Source: three-view drawing plus pictorial views. Frame: mm from the lowest corner of the part. A direction names the side the tool comes from. Coordinates: 2 decimals unless noted, no trailing zeros. Loops run counter-clockwise (first coordinate to the right, second up) from the corner with the lowest first, then second, coordinate; pieces in that order, holes last. Notation, with made-up numbers: (-5.5, 77.25) - (43.5, 77.25) arc R37 ccw to (43.5, 114.25) - close; hole circle Ø6 at (-23, -3.75). An arc over 180 degrees is marked (long way). Return JSON: item names as keys, results as strings.
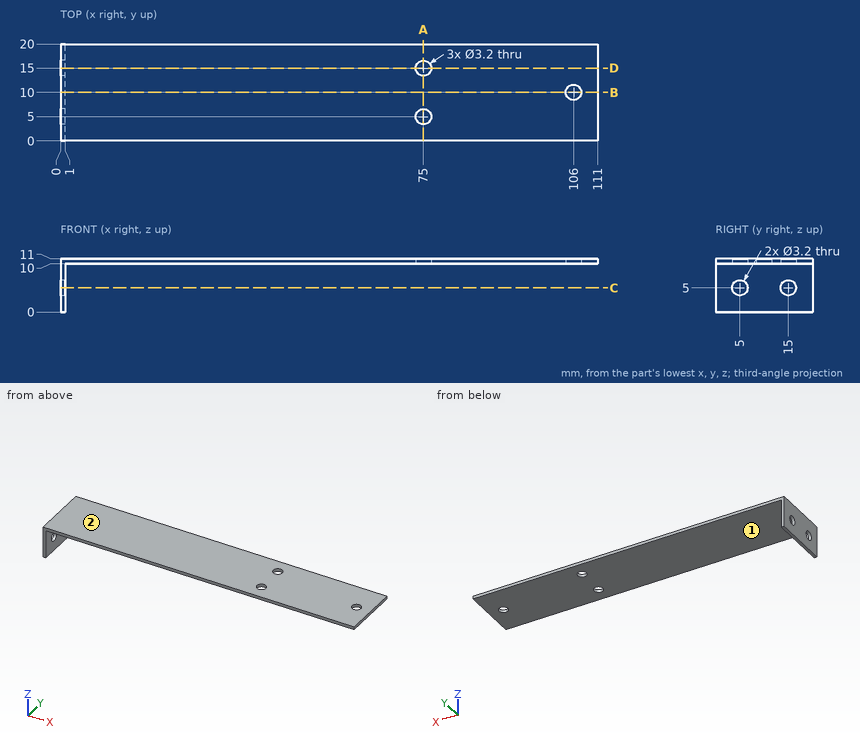
Item 1: Section query C-C, the plane z = 5. Return loops of the section in (x, y), and give its area (3 significant figures).
Worked out:
{"outline": "(0, 0) - (1, 0) - (1, 3.4) - (0, 3.4) - close; (0, 6.6) - (1, 6.6) - (1, 13.4) - (0, 13.4) - close; (0, 16.6) - (1, 16.6) - (1, 20) - (0, 20) - close", "area": "13.6 mm^2"}
Item 2: Reachability of the marked faces 1 and 2 from +Z, -Z, +X, -X, +Y, -Y: full face, straight path, thin tool, end or side. Return the list, or none.
Worked out:
{"face 1": "-Z, +X, +Y, -Y", "face 2": "+Z, +X, -X, +Y, -Y"}
Item 3: Ray query, probe 1 along Y at (x, z) = (0.45, 5); probe 2 along Y at (x, z) = (106, 10.2); probe 3 along X at (y, z) = (10, 10.7). Return the intervals inside material, ascending. Write a range as from..to.
Worked out:
{"probe 1": "0..3.4, 6.6..13.4, 16.6..20", "probe 2": "0..8.4, 11.6..20", "probe 3": "0..104.4, 107.6..111"}
Item 4: First-contact query: pin 1 Ø5 at (y, z) = (14.5, 6) entering from +X; pin 2 Ø4 at (x, y) = (12, 5.5) entering from -Z; pin 3 Ø3 at (x, y) = (75, 5) entering from -Z. Flat tips, straight axial feed; report the tip coordinate or a pass-through.
Worked out:
{"pin 1": "x = 1", "pin 2": "z = 10", "pin 3": "through"}
Item 5: Section query D-D, the plane y = 15. Return loops of the section in (x, z).
Worked out:
{"outline": "(0, 0) - (1, 0) - (1, 3.4) - (0, 3.4) - close; (0, 6.6) - (1, 6.6) - (1, 10) - (73.4, 10) - (73.4, 11) - (0, 11) - close; (76.6, 10) - (111, 10) - (111, 11) - (76.6, 11) - close"}
Item 6: Section query A-A, the plane x = 75. Return loops of the section in (y, z), and give its area (3 significant figures).
Worked out:
{"outline": "(0, 10) - (3.4, 10) - (3.4, 11) - (0, 11) - close; (6.6, 10) - (13.4, 10) - (13.4, 11) - (6.6, 11) - close; (16.6, 10) - (20, 10) - (20, 11) - (16.6, 11) - close", "area": "13.6 mm^2"}
Item 7: Section query B-B, the plane y = 10. Return loops of the section in (x, z).
Worked out:
{"outline": "(0, 0) - (1, 0) - (1, 10) - (104.4, 10) - (104.4, 11) - (0, 11) - close; (107.6, 10) - (111, 10) - (111, 11) - (107.6, 11) - close"}
